```python
from build123d import *

# Parameters (mm, degrees)
CUT_EXTRUDE1_DEPTH      = 13
CUT_EXTRUDE1_DEPTH_BACK = 13


with BuildPart() as part:
    # Sketch1 → Revolve1 (revolve)
    with BuildSketch(Plane(origin=(0, 0, 0), x_dir=(0, 0, -1), z_dir=(1, 0, 0))):
        with BuildLine():
            Line((-5.05, 8.746856578), (-12, 8.746856578))
            Line((-12, 8.746856578), (-12, -12))
            Line((-12, -12), (0, -12))
            Line((0, -12), (0, -10.1))
            ThreePointArc((0, -10.1), (-9.755850846, -2.614072356), (-5.05, 8.746856578))
        make_face()
    revolve(axis=Axis((0, -12, 0), (0, 1, 0)))

    # Sketch2 → Cut-Extrude1 (cut, two sides)
    with BuildSketch(Plane(origin=(0, 0, 0), x_dir=(0, 0, -1), z_dir=(1, 0, 0))) as cut_extrude1_sk:
        Polygon((-6.492154858, 7.737048876), (9.946558305, -1.753846594), (12, -2.93940171), (12, 8.746856578), (-12, 8.746856578), (-12, 7.737048876), align=None)
    extrude(amount=CUT_EXTRUDE1_DEPTH, mode=Mode.SUBTRACT)
    extrude(cut_extrude1_sk.sketch, amount=-CUT_EXTRUDE1_DEPTH_BACK, mode=Mode.SUBTRACT)


solid = part.part
```
Here's how the part is built. I have some questions about the finished solid (model axes, mm). Round coordinates to 2 decimals unless told otherwise and drop trailing zeros. Loops run counter-clockwise (first coordinate to the right, second up) from the corner with the lowest first, then second, coordinate; pieces in that order, holes last. Notation, with made-up numbers: (7.5, -17.5) -> (66.5, -17.5) arc R22 cw to (66.5, 12.5) -> close; hole circle Ø8 at (-29, 57). An arc over 180 degrees is marked (long way). Answer as CSV lines item,"result". Start each with the question number.
1. I need wall thicknesses on probe 1 along X at (y, z) = (6, 4.5); probe 2 along Z at (x, y) = (4.75, -2.25); probe 3 along X at (y, z) = (-0.75, 0). Which ranges of each line are inside material? Lowest first, please. Write a range as from..to.
2. Imagine slicing it at C-C on y = -5. Write out the boundary of the cut face in (x, z), plus the area to 3 significant figures.
3. I'm going to push flat-ended pins straight in: P1, Ø1, axis at x = 7, z = -9, coming from the +Y side; P2, Ø1, axis at y = -6.5, z = 6.5, coming from the +X side; P3, Ø4, axis at x = -7, y = 2, coming from the +Z side. Where does each tip first touch, or does it pass through?
4. Imagine slicing it at D-D on z = 0. Write out the boundary of the cut face in (x, y), plus the area to 3 significant figures.
5. Imagine slicing it at A-A on z = -3. Write out the boundary of the cut face in (x, y), plus the area to 3 significant figures.
6. Imagine slicing it at B-B on y = 3. Write out the boundary of the cut face in (x, z), plus the area to 3 significant figures.
Solution:
1,probe 1,"-11.12..-6.76, 6.76..11.12"
1,probe 2,"-10.81..-8.62, 8.62..11.02"
1,probe 3,"-12..-10.07, 10.07..12"
2,outline,"circle Ø24 at (0, 0); hole circle Ø17.55 at (0, 0)"
2,area,"210 mm²"
3,P1,"y = -0.92"
3,P2,"x = 10.39"
3,P3,"z = 10.91"
4,outline,"(-12, -12) -> (12, -12) -> (12, 3.99) -> (9.28, 3.99) arc R10.1 cw (long way) to (-9.28, 3.99) -> (-12, 3.99) -> close"
4,area,"145 mm²"
5,outline,"(-11.62, -12) -> (11.62, -12) -> (11.62, 2.26) -> (9.38, 2.26) arc R9.64 cw (long way) to (-9.38, 2.26) -> (-11.62, 2.26) -> close"
5,area,"142 mm²"
6,outline,"(-11.88, -1.71) -> (-9.49, -1.71) arc R9.64 cw (long way) to (9.49, -1.71) -> (11.88, -1.71) arc R12 ccw (long way) to start"
6,area,"88.2 mm²"
